Autodesk Inventor part; units mm, degrees
ref_plane "YZ Plane" through (0, 0, 0) normal (1, 0, 0) x (0, 1, 0)
ref_plane "XZ Plane" through (0, 0, 0) normal (0, 1, 0) x (-1, 0, 0)
ref_plane "XY Plane" through (0, 0, 0) normal (0, 0, 1) x (1, 0, 0)
sketch "Szkic1" plane through (0, 0, 0) normal (0, 0, 1) x (1, 0, 0)
  line L0 (0, 0) -> (10, 0)
  line L1 (10, 0) -> (10, 50)
  line L2 (10, 50) -> (0, 50)
  line L3 (0, 50) -> (0, 0)
  dimension "d0" = 50
  dimension "d1" = 10
extrude "Płyta1" add sketch "Szkic1" along normal blind 5
sketch "Szkic3" plane through (10, 5, 0) normal (0, -1, 0) x (1, 0, 0)
  line L0 (-10, 0) -> (0, 0)
  line L1 (0, 0) -> (0, 50)
  line L2 (0, 50) -> (-10, 50)
  line L3 (-10, 50) -> (-10, 0)
edge flange "Kołnierz1" height 50 angle 90 thickness 5 bend radius 5 thickness toward (0, -1, 0) relief tear relief width 5 relief depth 2.5 edges at (5, 0, 5) wall of the first edge with corners at (0, 5, 0) (10, 5, 0) (10, 5, 50) (0, 5, 50)
bend "Gięcie1"
corner "Narożnik1"
sketch "Szkic2" plane through (0, 0, 5) normal (0, 0, 1) x (1, 0, 0)
  line L0 (0, 0) -> (0, 50) construction
  line L1 (10, 50) -> (10, 0) construction
  arc A0 (10, 45) -> (0, 45) centre (5, 45) ccw
  line L2 (5, 23.75) -> (5.65, 23.75) construction
  point P0 (5, 42.5)
  point P1 (5, 5)
  point P2 (0, 5)
  point P3 (10, 5)
  dimension "d5" = 5
  dimension "d6" = 5
  dimension "d7" = 2.5
hole "Otwór4" at (5, 42.5, 5) at (5, 23.75, 5) direction (0, 0, -1) diameter 5 end through all
fillet "Zaokrąglenie2" radius 5 4 edges at (0, 2.5, 50) (10, 2.5, 50) (10, 50, 2.5) (0, 50, 2.5)
equation "\"d45\" = Grubość"
equation "\"d23\" = SzerokośćGięciaPodcięcia"
equation "\"d24\" = GłębokośćGięciaPodcięcia"
equation "\"d25\" = MinimalnaPozostałość"
equation "\"d26\" = PromieńGięcia"
equation "\"d29\" = PromieńGięcia"
equation "\"d30\" = RozmiarPodcięciaNarożnika"
equation "\"d31\" = Wielk_odstępu"
equation "\"d32\" = Rozmiar_promienia_Jacobiego"
equation "\"PromieńGięcia\" = Grubość"
equation "\"SzerokośćGięciaPodcięcia\" = Grubość"
equation "\"GłębokośćGięciaPodcięcia\" = 0.5 * Grubość"
equation "\"PromieńPrzejścia\" = PromieńGięcia"
equation "\"Rozmiar_promienia_Jacobiego\" = PromieńGięcia"
equation "\"Wielk_odstępu\" = Grubość"
equation "\"d2\" = PromieńGięcia"
properties part number "Pręt_łączący" material "Stal nierdzewna"
Work out the finished part from the listing and answer in its coordinate system (mm). A direction names the side the tool comes from. Round coordinates to 2 decimals unless told otherwise and drop trailing zeros. Write each loop counter-clockwise with the first axis right and the second up, starting at its lowest first coordinate (ties: lowest second). Pieces come first, ordered by that corner, then holes. Notation, with made-up numbers: (83, 3.5) - (120, 3.5) arc R8 ccw to (120, 10.5) - close; hole circle Ø9 at (40, 71.25). An arc over 180 degrees is marked (long way). Return JSON: item names as keys, results as strings. Group by question number.
Q1. The part is cut by section C-C on y = 41. Write down the section's boundary in (x, z), then the cut area to 3 significant figures.
Q2. The mould has two halves that part along Y. Classify faces 1 (the cylindrical face through (4.89, 26.248, 2.465)), 2 (the cylindrical face through (2, 2, 49)), 3 (the cylindrical face through (5.07, 2.85, 3.01)), 4 (the cylindrical face through (9, 48, 3)): released by +Y, released by -Y, zero draft, split by the parting line, or undercut.
Q3. The part is cut by section D-D on z = 32.5. Write down the section's boundary in (x, y), then the cut area to 3 significant figures.
Q4. The part is cut by section B-B on x = 5.75. Write down the section's boundary in (y, z), then the cut area to 3 significant figures.
Q5. The part is cut by section A-A on y = 23.75. Write down the section's boundary in (x, z).
Q6. Each of these flat-tipped pins is pushed along its axis until it touches: pin 1 Ø3 at (x, y) = (3, 30) entering from +Z; pin 2 Ø5 at (x, z) = (5, 37.5) entering from +Y; pin 3 Ø5 at (y, z) = (5.5, 36.5) entering from +X; pin 4 Ø4 at (x, y) = (5, 8.5) entering from +Z. Where does it stop, or does it pass through?
Q7. Find the intervals of material crossed by L1, parallel to X at y = 23.75, z = 2.55; L2, parallel to Y at x = 9, z = 27.5, in increasing order.
Q8. For faces 5 (the flat face through (5, 30, 5)), 6 (the flat face through (5, 0, 30)), determine the directions among +Z, -Z, +X, -X, +Y, -Y from which every point of the face is accessible in a straight line to the end or side of a thin tool.
Solved:
{
 "1": {"outline": "(0, 0) - (3, 0) - (3, 5) - (0, 5) - close; (7, 0) - (10, 0) - (10, 5) - (7, 5) - close", "area": "30.0 mm²"},
 "2": {"face 1": "undercut", "face 2": "zero draft", "face 3": "released by -Y", "face 4": "released by +Y"},
 "3": {"outline": "(0, 0) - (10, 0) - (10, 5) - (0, 5) - close", "area": "50.0 mm²"},
 "4": {"outline": "(0, 10) arc R10 ccw to (10, 0) - (21.37, 0) - (21.37, 5) - (10, 5) arc R5 cw to (5, 10) - (5, 49.94) - (0, 49.94) - close; (26.13, 0) - (40.12, 0) - (40.12, 5) - (26.13, 5) - close; (44.88, 0) - (49.94, 0) - (49.94, 5) - (44.88, 5) - close", "area": "411 mm²"},
 "5": {"outline": "(0, 0) - (2.5, 0) - (2.5, 5) - (0, 5) - close; (7.5, 0) - (10, 0) - (10, 5) - (7.5, 5) - close"},
 "6": {"pin 1": "z = 5", "pin 2": "y = 5", "pin 3": "x = 10", "pin 4": "z = 6.43"},
 "7": {"L1": "0 to 2.5, 7.5 to 10", "L2": "0 to 5"},
 "8": {"face 5": "+Z, +X, -X, +Y", "face 6": "+Z, -Z, +X, -X, -Y"}
}
